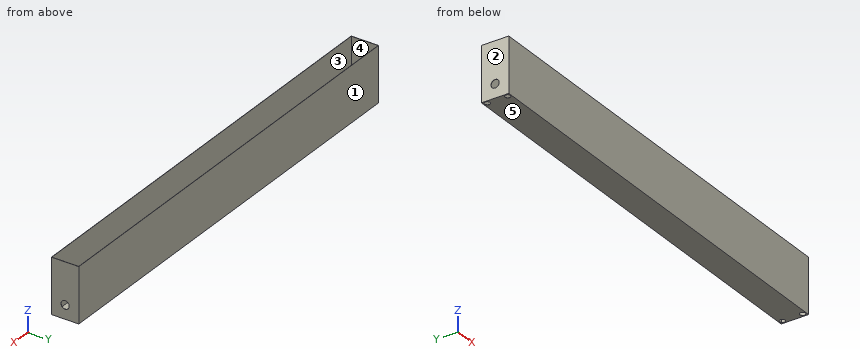
from build123d import *

# Parameters (mm, degrees)
F0_W     = 1600
F0_H     = 100
F1_DEPTH = 200
F2_T     = -1
F5_D     = 20
F8_D     = 30


# Not quite as in the source:
# - the program builds the solid bodies; features that only make, move or delete a surface that nothing else refers to are left out


with BuildPart() as f1:
    # F0 (on Top) → F1 (new body)
    with BuildSketch(Plane.XY):
        Rectangle(F0_W, F0_H)
    extrude(amount=F1_DEPTH)

    # F2
    f2_openings = [f1.faces().sort_by_distance(p)[0] for p in [
        (0, 0, 200),
    ]]
    offset(amount=F2_T, openings=f2_openings)

    # F5 (through all)
    with Locations(Plane.XY.offset(1)):
        with Locations((787, 37), (787, -37), (-787, 37), (-787, -37)):
            Hole(F5_D / 2)

    # F8 (through all)
    with Locations(Plane(origin=(-800, 0, 0), x_dir=(0, -1, 0), z_dir=(-1, 0, 0))):
        with Locations((0, 50)):
            Hole(F8_D / 2)


solid = f1.part
The listing builds one solid part. Answer for the finished solid, in the listing's coordinates (mm). Face numbers are marked on the shaded views. A direction names the side the tool comes from. Round coordinates to 2 decimals unless told otherwise and drop trailing zeros. Write each loop counter-clockwise with the first axis right and the second up, starting at its lowest first coordinate (ties: lowest second). Pieces come first, ordered by that corner, then holes. Notation, with made-up numbers: (12, -32) - (49, -32) arc R11 ccw to (49, -17) - close; hole circle Ø11 at (50.5, 59). An arc over 180 degrees is marked (long way). Use one line per item in the form item = value. Start each with the question number.
Item 1: A flat-ended cylindrical pin translates along its axis: pin 1 Ø1 at (x, y) = (490, -35.5) entering from +Z. Find the tip coordinate at first contact, or state that the pin passes through.
Item 2: A cutting plane is placed at B-B (x = 595). Write down the section's boundary in (y, z), plus the area to 3 significant figures.
Item 3: Find the intervals of material crossed by line 1 (Y direction, x = 787, z = 0.4); line 2 (X direction, y = -37.5, z = 78.5); line 3 (Y direction, x = 191, z = 29.5), in increasing order. Write a range as [from, to].
Item 4: A cutting plane is placed at A-A (z = 50). Write down the section's boundary in (x, y), plus the area to 3 significant figures.
Item 5: A tool of negligible diameter and unlimited length cuts with its end or side. For the marked faces 4 and 5, from which of +Z, -Z, +X, -X, +Y, -Y can it reach the whole face along a straight path? Write none if from no direction.
Item 6: Determine the mould class of the marked faces 1, 2 and 3 for opening direction X: +X half, -X half, draft (parallel to the pull), parting line (faces both ways), or undercut.
The answers:
q1.pin_1 = 1
q2.outline = (-50, 0) - (50, 0) - (50, 200) - (49, 200) - (49, 1) - (-49, 1) - (-49, 200) - (-50, 200) - close
q2.area = 498 mm^2
q3.line_1 = [-50, -47], [-27, 27], [47, 50]
q3.line_2 = [-800, -799], [799, 800]
q3.line_3 = [-50, -49], [49, 50]
q4.outline = (-800, -50) - (800, -50) - (800, -15) - (799, -15) - (799, -49) - (-799, -49) - (-799, -15) - (-800, -15) - close; (-800, 15) - (-799, 15) - (-799, 49) - (799, 49) - (799, 15) - (800, 15) - (800, 50) - (-800, 50) - close
q4.area = 3,340 mm^2
q5.face_4 = +Z
q5.face_5 = -Z, +X, -X, +Y, -Y
q6.face_1 = draft
q6.face_2 = -X half
q6.face_3 = undercut
